Input: part model. Units: mm. Frame: model coordinates. A direction names the side the tool comes from. Coordinates: 2 decimals unless noted, no trailing zeros. Loops run counter-clockwise (first coordinate to the right, second up) from the corner with the lowest first, then second, coordinate; pieces in that order, holes last.
```python
from build123d import *

# Parameters (mm, degrees)
SKETCH_1_R          = 9
EXTRUDE_1_DEPTH     = 20
CUT_EXTRUDE_1_DEPTH = 7
SKETCH_3_R          = 7
CUT_EXTRUDE_2_DEPTH = 13
CUT_EXTRUDE_3_DEPTH = 13
CUT_EXTRUDE_4_DEPTH = 13


with BuildPart() as part:
    # 草图1 → 凸台-拉伸1 (new body)
    with BuildSketch(Plane(origin=(0, 0, 0), x_dir=(1, 0, 0), z_dir=(0, 1, 0))):
        with Locations(Location((0, 0, 0), (0, 0, 270))):
            Circle(SKETCH_1_R)
    extrude(amount=EXTRUDE_1_DEPTH)

    # 草图2 → 切除-拉伸1 (cut)
    with BuildSketch(Plane(origin=(0, 0, 0), x_dir=(-1, 0, 0), z_dir=(0, -1, 0))):
        with BuildLine():
            Line((2.121320344, 1.75), (-2.121320344, 1.75))
            ThreePointArc((-2.121320344, 1.75), (-2.75, 0), (-2.121320344, -1.75))
            Line((-2.121320344, -1.75), (2.121320344, -1.75))
            ThreePointArc((2.121320344, -1.75), (2.75, 0), (2.121320344, 1.75))
        make_face()
    extrude(amount=-CUT_EXTRUDE_1_DEPTH, mode=Mode.SUBTRACT)

    # 草图3 → 切除-拉伸2 (cut)
    with BuildSketch(Plane(origin=(0, 20, 0), x_dir=(1, 0, 0), z_dir=(0, 1, 0))):
        with Locations(Location((0, 0, 0), (0, 0, 270))):
            Circle(SKETCH_3_R)
    extrude(amount=-CUT_EXTRUDE_2_DEPTH, mode=Mode.SUBTRACT)

    # 草图8 → 切除-拉伸3 (cut)
    with BuildSketch(Plane(origin=(0, 20, 0), x_dir=(1, 0, 0), z_dir=(0, 1, 0))):
        with BuildLine():
            Line((-1.5, -10.84621088), (-1.5, 10.935737737))
            ThreePointArc((-1.5, 10.935737737), (0, 12.435737737), (1.5, 10.935737737))
            Line((1.5, 10.935737737), (1.5, -10.84621088))
            ThreePointArc((1.5, -10.84621088), (0, -12.34621088), (-1.5, -10.84621088))
        make_face()
    extrude(amount=-CUT_EXTRUDE_3_DEPTH, mode=Mode.SUBTRACT)

    # 草图9 → 切除-拉伸4 (cut)
    with BuildSketch(Plane(origin=(0, 20, 0), x_dir=(1, 0, 0), z_dir=(0, 1, 0))):
        with BuildLine():
            Line((-9.142857143, 1.5), (9.171653543, 1.5))
            ThreePointArc((9.171653543, 1.5), (10.671653543, 0), (9.171653543, -1.5))
            Line((9.171653543, -1.5), (-9.142857143, -1.5))
            ThreePointArc((-9.142857143, -1.5), (-10.642857143, 0), (-9.142857143, 1.5))
        make_face()
    extrude(amount=-CUT_EXTRUDE_4_DEPTH, mode=Mode.SUBTRACT)


solid = part.part
```
Item 1: Contact query for flat-ended pins moving along their axis: P1, Ø5, axis at x = 0, z = 3, coming from the +Y side; P2, Ø3.5, axis at x = 1, y = 4.5, coming from the +Z side; P3, Ø8, axis at x = -6, y = 2, coming from the -Z side; P4, Ø8, axis at y = 14.5, z = -0.5, coming from the +X side. Output: stop coordinate, or through.
Result:
P1: stops at y = 7
P2: stops at z = 9
P3: stops at z = -8.77
P4: stops at x = 8.87
Item 2: Section query A-A (y = 11.75). Output: boundary loops of the cut face in (x, z).
Result:
outline: (-8.87, -1.5) arc R9 ccw to (-1.5, -8.87) - (-1.5, -6.84) arc R7 cw to (-6.84, -1.5) - close; (-8.87, 1.5) - (-6.84, 1.5) arc R7 cw to (-1.5, 6.84) - (-1.5, 8.87) arc R9 ccw to start; (1.5, -8.87) arc R9 ccw to (8.87, -1.5) - (6.84, -1.5) arc R7 cw to (1.5, -6.84) - close; (1.5, 6.84) arc R7 cw to (6.84, 1.5) - (8.87, 1.5) arc R9 ccw to (1.5, 8.87) - close
Item 3: Section query C-C (z = 0). Output: boundary loops of the cut face in (x, y), then the cut area to 3 significant figures.
Result:
outline: (-9, 0) - (-2.75, 0) - (-2.75, 7) - (-9, 7) - close; (2.75, 0) - (9, 0) - (9, 7) - (2.75, 7) - close
area: 87.5 mm2
Item 4: Section query D-D (y = 3.25). Output: boundary loops of the cut face in (x, z).
Result:
outline: circle Ø18 at (0, 0); hole (-2.12, -1.75) - (2.12, -1.75) arc R2.75 ccw to (2.12, 1.75) - (-2.12, 1.75) arc R2.75 ccw to start
Item 5: Line query: L1, parallel to Y at x = 4.25, z = 1.5; L2, parallel to Z at x = 1.75, y = 6.5; L3, parallel to Z at x = -0.75, y = 3. Output: solid intervals per line, ascending.
Result:
L1: y = 0 to 7
L2: z = -8.83 to -1.75, 1.75 to 8.83
L3: z = -8.97 to -1.75, 1.75 to 8.97
Item 6: Mould query, pull axis X, two halves, no side actions, for faces 1 (the face through (-3.447, 9.86, 8.314)), 2 (the face through (8, 14, -1.5)), 3 (the face through (-4.9, 13.6, -5)). Classes: +X half, -X half, draft (parallel to the pull), parting line (faces both ways), or undercut.
Result:
face 1: parting line
face 2: draft
face 3: undercut
Item 7: Reachability of faces 4 (the face through (5.2, 20, 5.4)), 5 (the face through (0, 3, -1.75)), 6 (the face through (-1.5, 14, 8)), 7 (the face through (-8, 14, 1.5)), 8 (the face through (4.9, 13.6, 5)) from +Z, -Z, +X, -X, +Y, -Y: full face, straight path, thin tool, end or side. Return the list, or none.
Result:
face 4: +Z, -Z, +X, -X, +Y
face 5: +Y, -Y
face 6: +Z, -Z, +Y
face 7: +X, -X, +Y
face 8: +Y
Item 8: Section query B-B (x = 0). Output: boundary loops of the cut face in (y, z).
Result:
outline: (0, -9) - (7, -9) - (7, -1.75) - (0, -1.75) - close; (0, 1.75) - (7, 1.75) - (7, 9) - (0, 9) - close
